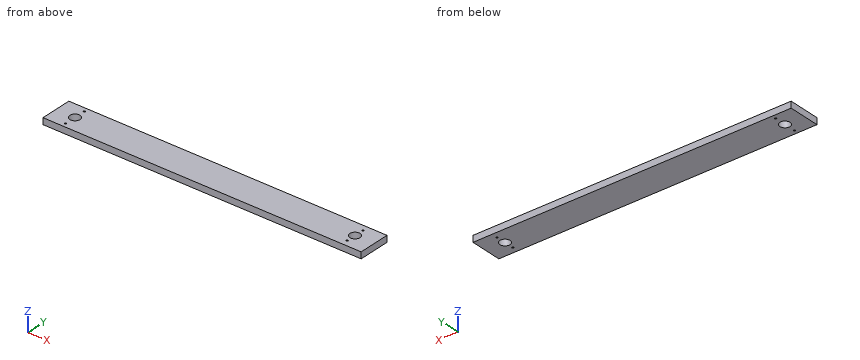
```python
from build123d import *

# Parameters (mm, degrees)
F0_W     = 250
F0_H     = 25
F1_DEPTH = 5
F3_D     = 1.4732
F4_D     = 1.4732
F5_D     = 1.4732
F6_D     = 8


with BuildPart() as f1:
    # F0 (on Top) → F1 (new body)
    with BuildSketch(Plane.XY):
        with Locations((11.708578, -66.683836)):
            Rectangle(F0_W, F0_H)
    extrude(amount=F1_DEPTH)

    # F3 (through all)
    with Locations(Plane.XY.offset(5)):
        with Locations((-98.291422, -57.590636)):
            Hole(F3_D / 2)

    # F4 (through all)
    with Locations(Plane.XY.offset(5)):
        with Locations((-98.291422, -75.777036)):
            Hole(F4_D / 2)

    # F5 (through all)
    with Locations(Plane.XY.offset(5)):
        with Locations((121.708578, -59.063836), (121.708578, -74.303836)):
            Hole(F5_D / 2)

    # F6 (through all)
    with Locations(Plane.XY.offset(5)):
        with Locations((-98.291422, -66.683836), (121.708578, -66.683836)):
            Hole(F6_D / 2)


solid = f1.part
```
Here's how the part is built. I have some questions about the finished solid (model axes, mm). Round coordinates to 2 decimals unless told otherwise and drop trailing zeros. Order: outer loops, then holes, each group sorted by start corner. A loop starts at its lowest first (then second) coordinate and runs counter-clockwise, first axis right, second up. Notation, with made-up numbers: (-26, -18) -> (-13, -18) arc R16 cw to (-13, 12) -> close; hole circle Ø2 at (-20, 72). An arc over 180 degrees is marked (long way). Use a Markdown table: item, result. Add a question column.
(1) Suppose I cut it at A-A, the plane z = 2.05. Please give me the cut outline in (x, y), and give its area (3 significant figures).
(2) For pin 1 Ø6.5 at (x, y) = (-98.29, -66.68) entering from +Z; pin 2 Ø1.7 at (x, y) = (-98.29, -57.59) entering from -Z, each with a flat end and sliding along its axis, tell me the tip position at first contact or that it passes through.
(3) I need wall thicknesses on line 1 along X through (y, z) = (-66, 3.9); line 2 along X through (y, z) = (-67.75, 0.35); line 3 along Y through (x, z) = (123.5, 0.5). Which ranges of each line are inside material? Lowest first, please.
Verdict:
| question | item | result |
|---|---|---|
| 1 | outline | (-113.29, -79.18) -> (136.71, -79.18) -> (136.71, -54.18) -> (-113.29, -54.18) -> close; hole circle Ø8 at (-98.29, -66.68); hole circle Ø1.47 at (-98.29, -75.78); hole circle Ø1.47 at (-98.29, -57.59); hole circle Ø8 at (121.71, -66.68); hole circle Ø1.47 at (121.71, -74.3); hole circle Ø1.47 at (121.71, -59.06) |
| 1 | area | 6,140 mm2 |
| 2 | pin 1 | through |
| 2 | pin 2 | z = 0 |
| 3 | line 1 | -113.29 to -102.23, -94.35 to 117.77, 125.65 to 136.71 |
| 3 | line 2 | -113.29 to -102.15, -94.44 to 117.85, 125.56 to 136.71 |
| 3 | line 3 | -79.18 to -70.26, -63.11 to -54.18 |
